```python
from build123d import *

# Parameters (mm, degrees)
F0_R     = 1.179689
F1_DEPTH = 2.54


with BuildPart() as f1:
    # F0 (on Right) → F1 (new body)
    with BuildSketch(Plane.YZ):
        Polygon((2.86521, 4.212468), (-2.610088, 4.212468), (-2.433466, 0.326772), (2.86521, 0.326772), align=None)
        Polygon((2.86521, 0.326772), (-2.433466, 0.326772), (-2.433466, -4.265413), (1.098984, -4.08879), align=None)
        with Locations((0.215872, -1.377823)):
            Circle(F0_R, mode=Mode.SUBTRACT)
    extrude(amount=F1_DEPTH)


solid = f1.part
```
Input: part model. Units: mm. Frame: model coordinates. A direction names the side the tool comes from. Round coordinates to 2 decimals unless told otherwise and drop trailing zeros. Loops run counter-clockwise (first coordinate to the right, second up) from the corner with the lowest first, then second, coordinate; pieces in that order, holes last.
1) Pin query (flat end, axial travel): pin 1 (1.4 mm diameter, centred on y = 0.22, z = -1.38, fed in from -X); pin 2 (1.3 mm diameter, centred on x = 1, z = -2, fed in from -Y); pin 3 (1.5 mm diameter, centred on x = 0.5, y = -1.5, fed in from -Z). Return the tip coordinate at first contact, or that it passes through.
Ans:
pin 1: passes through
pin 2: stops at y = -2.43
pin 3: stops at z = -4.26
2) Material intervals for line 1 (Y direction, x = 0.9, z = 3); line 2 (Z direction, x = 1.4, y = 0); line 3 (Y direction, x = 0.2, z = -0.5), sorted ascending.
Ans:
line 1: y = -2.55 to 2.87
line 2: z = -4.14 to -2.54, -0.22 to 4.21
line 3: y = -2.43 to -0.57, 1 to 2.53
3) Set-up query: faces 4 (the flat face through (1, -2.433, -2)), 5 (the flat face through (0, 0, 0)). Return all of +Z, -Z, +X, -X, +Y, -Y with unobstructed straight access to the full face (end or side cutting, diameter ignored); none if empty.
Ans:
face 4: -Z, +X, -X, -Y
face 5: +Z, -Z, -X, +Y, -Y
4) Section query C-C on z = 2. Return the cut outline in (x, y).
Ans:
outline: (0, -2.51) - (2.54, -2.51) - (2.54, 2.87) - (0, 2.87) - close
5) Pull-direction query (Y, two-part tool) for faces 1 (the flat face through (1.25, -0.69, -4.18)), 2 (the cylindrical face through (1.25, -0.04, -2.53)), 3 (the flat face through (1.252, -2.523, 2.297)); classes: released by +Y, released by -Y, zero draft, split by the parting line, or undercut.
Ans:
face 1: released by +Y
face 2: undercut
face 3: released by -Y
6) Section query B-B on x = 1.4. Return the cut outline in (y, z), plus the area to 3 significant figures.
Ans:
outline: (-2.61, 4.21) - (-2.43, 0.33) - (-2.43, -4.27) - (1.1, -4.09) - (2.87, 0.33) - (2.87, 4.21) - close; hole circle Ø2.36 at (0.22, -1.38)
area: 36.4 mm2
7) Section query D-D on z = 0.5. Return the cut outline in (x, y).
Ans:
outline: (0, -2.44) - (2.54, -2.44) - (2.54, 2.87) - (0, 2.87) - close
8) Section query A-A on y = 1.2. Return the cut outline in (x, z), plus the area to 3 significant figures.
Ans:
outline: (0, -3.84) - (2.54, -3.84) - (2.54, -2.03) - (0, -2.03) - close; (0, -0.73) - (2.54, -0.73) - (2.54, 4.21) - (0, 4.21) - close
area: 17.1 mm2
